Here's how the part is built. I have some questions about the finished solid (model axes, mm). A direction names the side the tool comes from. Round coordinates to 2 decimals unless told otherwise and drop trailing zeros. Order: outer loops, then holes, each group sorted by start corner. A loop starts at its lowest first (then second) coordinate and runs counter-clockwise, first axis right, second up.
```python
from build123d import *

# Parameters (mm, degrees)
SKETCH1_W           = 130
SKETCH1_H           = 73.5
BOSS_EXTRUDE1_DEPTH = 5
SKETCH2_R           = 24.718
SKETCH2_R_2         = 18.718
CUT_EXTRUDE1_DEPTH  = 2
FILLET1_R           = 3.25
SKETCH3_W           = 10
SKETCH3_H           = 73.5
BOSS_EXTRUDE2_DEPTH = 11
SKETCH4_R           = 2
CUT_EXTRUDE2_DEPTH  = 90.059320119
SKETCH5_R           = 16.5
CUT_EXTRUDE3_DEPTH  = 89.580824674
SKETCH7_W           = 150
SKETCH7_H           = 93.5
SKETCH7_R           = 16.5
SKETCH7_R_2         = 2
BOSS_EXTRUDE3_DEPTH = 2
SKETCH8_R           = 2
CUT_EXTRUDE5_DEPTH  = 90.328396941
SKETCH9_R           = 3.25
CUT_EXTRUDE6_DEPTH  = 6
SKETCH10_W          = 13
SKETCH10_H          = 150
BOSS_EXTRUDE4_DEPTH = 2
SKETCH11_W          = 13
SKETCH11_H          = 150
BOSS_EXTRUDE5_DEPTH = 2
SKETCH12_W          = 13
SKETCH12_H          = 97.5
BOSS_EXTRUDE6_DEPTH = 2
SKETCH13_W          = 13
SKETCH13_H          = 97.5
BOSS_EXTRUDE7_DEPTH = 2
SKETCH14_R          = 2.5
CUT_EXTRUDE7_DEPTH  = 93.057386993
CHAMFER1_SIZE       = 3


with BuildPart() as part:
    # Sketch1 → Boss-Extrude1 (new body)
    with BuildSketch(Plane(origin=(0, 0, 0), x_dir=(0, 0, -1), z_dir=(1, 0, 0))):
        Rectangle(SKETCH1_W, SKETCH1_H)
    extrude(amount=BOSS_EXTRUDE1_DEPTH)

    # Sketch2 → Cut-Extrude1 (cut)
    # profile 1 of 2: a face of its own
    with BuildSketch(Plane(origin=(5, 0, 0), x_dir=(0, 0, -1), z_dir=(1, 0, 0))):
        with Locations((28.125, 0)):
            Circle(SKETCH2_R)
        with Locations((28.125, 0)):
            Circle(SKETCH2_R_2, mode=Mode.SUBTRACT)
    # profile 2 of 2: a face of its own
    with BuildSketch(Plane(origin=(5, 0, 0), x_dir=(0, 0, -1), z_dir=(1, 0, 0))):
        with Locations(Location((-28.125, 0, 0), (0, 0, 180))):
            Circle(SKETCH2_R)
        with Locations(Location((-28.125, 0, 0), (0, 0, 180))):
            Circle(SKETCH2_R_2, mode=Mode.SUBTRACT)
    extrude(amount=-CUT_EXTRUDE1_DEPTH, mode=Mode.SUBTRACT)

    # Fillet1
    # the kernel refuses this fillet: 3.25 mm, written as the material it adds along each edge
    with BuildSketch(Plane(origin=(3, 0, -28.125), x_dir=(0, 0, -1), z_dir=(0, -1, 0))) as fillet1_piece_1:
        with BuildLine():
            CenterArc((21.718, 3.25), FILLET1_R, 270, 67.380135052)
            Line((21.718, 0), (21.718, -0.065))
            Line((21.718, -0.065), (24.718, -0.065))
            Line((24.718, -0.065), (24.783, 0))
            ThreePointArc((24.783, 0), (24.783, 1), (24.778, 1.975))
            Line((24.778, 1.975), (24.718, 2))
        make_face()
    revolve(axis=Axis((3, 0, -28.125), (1, 0, 0)))
    with BuildSketch(Plane(origin=(3, 0, -28.125), x_dir=(0, 0, -1), z_dir=(0, -1, 0))) as fillet1_piece_2:
        with BuildLine():
            CenterArc((21.718, 3.25), FILLET1_R, 202.619864948, 67.380135052)
            Line((18.718, 2), (18.658, 1.975))
            ThreePointArc((18.658, 1.975), (18.653, 1), (18.653, 0))
            Line((18.653, 0), (18.718, -0.065))
            Line((18.718, -0.065), (21.718, -0.065))
            Line((21.718, -0.065), (21.718, 0))
        make_face()
    revolve(axis=Axis((3, 0, -28.125), (1, 0, 0)))
    with BuildSketch(Plane(origin=(3, 0, 28.125), x_dir=(0, 0, 1), z_dir=(0, 1, 0))) as fillet1_piece_3:
        with BuildLine():
            CenterArc((21.718, 3.25), FILLET1_R, 270, 67.380135052)
            Line((21.718, 0), (21.718, -0.065))
            Line((21.718, -0.065), (24.718, -0.065))
            Line((24.718, -0.065), (24.783, 0))
            ThreePointArc((24.783, 0), (24.783, 1), (24.778, 1.975))
            Line((24.778, 1.975), (24.718, 2))
        make_face()
    revolve(axis=Axis((3, 0, 28.125), (1, 0, 0)))
    with BuildSketch(Plane(origin=(3, 0, 28.125), x_dir=(0, 0, 1), z_dir=(0, 1, 0))) as fillet1_piece_4:
        with BuildLine():
            CenterArc((21.718, 3.25), FILLET1_R, 202.619864948, 67.380135052)
            Line((18.718, 2), (18.658, 1.975))
            ThreePointArc((18.658, 1.975), (18.653, 1), (18.653, 0))
            Line((18.653, 0), (18.718, -0.065))
            Line((18.718, -0.065), (21.718, -0.065))
            Line((21.718, -0.065), (21.718, 0))
        make_face()
    revolve(axis=Axis((3, 0, 28.125), (1, 0, 0)))

    # Sketch3 → Boss-Extrude2 (add)
    with BuildSketch(Plane.ZY):
        Polygon((65, 36.75), (75, 36.75), (75, 46.75), (-75, 46.75), (-75, 36.75), (-65, 36.75), align=None)
        with Locations((70, 0)):
            Rectangle(SKETCH3_W, SKETCH3_H)
        Polygon((-65, -36.75), (-75, -36.75), (-75, -46.75), (75, -46.75), (75, -36.75), (65, -36.75), align=None)
        with Locations((-70, 0)):
            Rectangle(SKETCH3_W, SKETCH3_H)
    extrude(amount=-BOSS_EXTRUDE2_DEPTH)

    # Sketch4 → Cut-Extrude2 (cut, through all)
    with BuildSketch(Plane(origin=(11, 0, 0), x_dir=(0, 0, -1), z_dir=(1, 0, 0))):
        with Locations((-37.5, 41.75)):
            Circle(SKETCH4_R)
        with Locations((37.5, 41.75)):
            Circle(SKETCH4_R)
        with Locations((70, 20.875)):
            Circle(SKETCH4_R)
        with Locations(Location((-37.5, -41.75, 0), (0, 0, 180))):
            Circle(SKETCH4_R)
        with Locations(Location((37.5, -41.75, 0), (0, 0, 180))):
            Circle(SKETCH4_R)
        with Locations((70, -20.875)):
            Circle(SKETCH4_R)
        with Locations(Location((-70, 20.875, 0), (0, 0, 180))):
            Circle(SKETCH4_R)
        with Locations(Location((-70, -20.875, 0), (0, 0, 180))):
            Circle(SKETCH4_R)
    extrude(amount=-CUT_EXTRUDE2_DEPTH, mode=Mode.SUBTRACT)

    # Sketch5 → Cut-Extrude3 (cut, through all)
    with BuildSketch(Plane(origin=(5, 0, 0), x_dir=(0, 0, -1), z_dir=(1, 0, 0))):
        with Locations((-28.125, 0)):
            Circle(SKETCH5_R)
        with Locations((28.125, 0)):
            Circle(SKETCH5_R)
    extrude(amount=-CUT_EXTRUDE3_DEPTH, mode=Mode.SUBTRACT)

    # Sketch7 → Boss-Extrude3 (add)
    with BuildSketch(Plane.ZY):
        Rectangle(SKETCH7_W, SKETCH7_H)
        with Locations(Location((28.125, 0, 0), (0, 0, 180))):
            Circle(SKETCH7_R, mode=Mode.SUBTRACT)
        with Locations(Location((-28.125, 0, 0), (0, 0, 180))):
            Circle(SKETCH7_R, mode=Mode.SUBTRACT)
        with Locations(Location((-70, 20.875, 0), (0, 0, 180))):
            Circle(SKETCH7_R_2, mode=Mode.SUBTRACT)
        with Locations(Location((-70, -20.875, 0), (0, 0, 180))):
            Circle(SKETCH7_R_2, mode=Mode.SUBTRACT)
        with Locations((-37.5, -41.75)):
            Circle(SKETCH7_R_2, mode=Mode.SUBTRACT)
        with Locations((37.5, -41.75)):
            Circle(SKETCH7_R_2, mode=Mode.SUBTRACT)
        with Locations((70, -20.875)):
            Circle(SKETCH7_R_2, mode=Mode.SUBTRACT)
        with Locations((70, 20.875)):
            Circle(SKETCH7_R_2, mode=Mode.SUBTRACT)
        with Locations(Location((-37.5, 41.75, 0), (0, 0, 180))):
            Circle(SKETCH7_R_2, mode=Mode.SUBTRACT)
        with Locations(Location((37.5, 41.75, 0), (0, 0, 180))):
            Circle(SKETCH7_R_2, mode=Mode.SUBTRACT)
    extrude(amount=BOSS_EXTRUDE3_DEPTH)

    # Sketch8 → Cut-Extrude5 (cut, through all)
    with BuildSketch(Plane(origin=(11, 0, 0), x_dir=(0, 0, -1), z_dir=(1, 0, 0))):
        with Locations((11.37, 42.75)):
            Circle(SKETCH8_R)
        with Locations((20.07, 42.75)):
            Circle(SKETCH8_R)
        with Locations((11.37, -42.75)):
            Circle(SKETCH8_R)
        with Locations((20.07, -42.75)):
            Circle(SKETCH8_R)
        with Locations((71, 4.35)):
            Circle(SKETCH8_R)
        with Locations((71, -4.35)):
            Circle(SKETCH8_R)
    extrude(amount=-CUT_EXTRUDE5_DEPTH, mode=Mode.SUBTRACT)

    # Sketch9 → Cut-Extrude6 (cut)
    with BuildSketch(Plane(origin=(11, 0, 0), x_dir=(0, 0, -1), z_dir=(1, 0, 0))):
        with Locations((20.07, 42.75)):
            Circle(SKETCH9_R)
        with Locations((11.37, 42.75)):
            Circle(SKETCH9_R)
        with Locations((71, 4.35)):
            Circle(SKETCH9_R)
        with Locations((71, -4.35)):
            Circle(SKETCH9_R)
        with Locations((20.07, -42.75)):
            Circle(SKETCH9_R)
        with Locations((11.37, -42.75)):
            Circle(SKETCH9_R)
    extrude(amount=-CUT_EXTRUDE6_DEPTH, mode=Mode.SUBTRACT)

    # Sketch10 → Boss-Extrude4 (add)
    with BuildSketch(Plane(origin=(0, 46.75, 0), x_dir=(1, 0, 0), z_dir=(0, 1, 0))):
        with Locations((4.5, 0)):
            Rectangle(SKETCH10_W, SKETCH10_H)
    extrude(amount=BOSS_EXTRUDE4_DEPTH)

    # Sketch11 → Boss-Extrude5 (add)
    with BuildSketch(Plane.XZ.offset(46.75)):
        with Locations((4.5, 0)):
            Rectangle(SKETCH11_W, SKETCH11_H)
    extrude(amount=BOSS_EXTRUDE5_DEPTH)

    # Sketch12 → Boss-Extrude6 (add)
    with BuildSketch(Plane(origin=(0, 0, -75), x_dir=(-1, 0, 0), z_dir=(0, 0, -1))):
        with Locations((-4.5, 0)):
            Rectangle(SKETCH12_W, SKETCH12_H)
    extrude(amount=BOSS_EXTRUDE6_DEPTH)

    # Sketch13 → Boss-Extrude7 (add)
    with BuildSketch(Plane.XY.offset(75)):
        with Locations((4.5, 0)):
            Rectangle(SKETCH13_W, SKETCH13_H)
    extrude(amount=BOSS_EXTRUDE7_DEPTH)

    # Sketch14 → Cut-Extrude7 (cut, through all)
    with BuildSketch(Plane(origin=(11, 0, 0), x_dir=(0, 0, -1), z_dir=(1, 0, 0))):
        with Locations((71, 42.75)):
            Circle(SKETCH14_R)
        with Locations((-71, 42.75)):
            Circle(SKETCH14_R)
        with Locations((-71, -42.75)):
            Circle(SKETCH14_R)
        with Locations((71, -42.75)):
            Circle(SKETCH14_R)
    extrude(amount=-CUT_EXTRUDE7_DEPTH, mode=Mode.SUBTRACT)

    # Chamfer1
    chamfer1_edges = [part.edges().sort_by_distance(p)[0] for p in [
        (-2, -42.75, -68.5),
        (-2, -42.75, 73.5),
        (-2, 42.75, 73.5),
        (-2, 42.75, -68.5),
    ]]
    chamfer(chamfer1_edges, length=CHAMFER1_SIZE)


solid = part.part
```
1. If we mould it in two halves opening along Z, with no side actions, what happens to faces 3 (the flat face through (11, -40, 5)), 4 (the cylindrical face through (1.549, -44.702, -19.636))? For each: released by +Z, released by -Z, zero draft, split by the parting line, or undercut.
Evaluation:
face 3: zero draft
face 4: undercut
2. If we section it at A-A, the plane y = -29.5: Write out the boundary of the cut face in (x, z), and give its area (3 significant figures).
Evaluation:
outline: (-2, -77) - (11, -77) - (11, -65) - (5, -65) - (5, 65) - (11, 65) - (11, 77) - (-2, 77) - close
area: 1,220 mm2
3. If we section it at B-B, the plane x = 9: State how many separate pieces and enclosed holes the cut face has, and give its area (3 significant figures).
Evaluation:
separate pieces: 1
enclosed holes: 19
area: 5,080 mm2
4. On a 3-axis mill with a long thin cutter (end or side, diameter ignored), from which of +Z, -Z, +X, -X, +Y, -Y can I reach the whole of each face in a straight line? I mean faces 1 (the cylindrical face through (4.591, -20.274, 71.908)), 2 (the flat face through (8, -1, -65)). Say none if no direction works.
Evaluation:
face 1: +X, -X
face 2: +X
5. I need wall thicknesses on probe 1 along Z at (x, y) = (-0.5, -22); probe 2 along Y at (x, z) = (9, -46.5); probe 3 along Z at (x, y) = (6.5, 28). Which ranges of each line are inside material? Lowest first, please.
Evaluation:
probe 1: z = -77 to -71.65, -68.35 to 68.35, 71.65 to 77
probe 2: y = -48.75 to -36.75, 36.75 to 48.75
probe 3: z = -77 to -65, 65 to 77
6. I'm going to push flat-ended pins straight in: P1, Ø1.5, axis at y = -14, z = -7, coming from the +X side; P2, Ø6.5, axis at y = -42.75, z = 71, coming from the -X side; P3, Ø4.5, axis at y = -42.75, z = -71, coming from the -X side (3 decimals). Where does each tip first touch, or does it pass through?
Evaluation:
P1: stops at x = 5
P2: stops at x = 0.25
P3: passes through
